Could you check a few things on this drawing? It's one solid part, dimensions in mm from its lowest x, y, z. A direction names the side the tool comes from. Give positions to 0.01 mm unless a question says otherwise; leave off trailing zeros. Loops run counter-clockwise (first coordinate to the right, second up) from the corner with the lowest first, then second, coordinate; pieces in that order, holes last. Notation, with made-up numbers: (62.5, 15.25) - (83.5, 15.25) arc R37 cw to (83.5, 51.25) - close; hole circle Ø3 at (-28, 80). An arc over 180 degrees is marked (long way). Return JSON: item names as keys, results as strings. Group by question number.
(1) On a 3-axis mill with a long thin cutter (end or side, diameter ignored), from which of +Z, -Z, +X, -X, +Y, -Y can I reach the whole of each face in a straight line? I mean the marked faces 1 and 2. Say none if no direction works.
(2) If we section it at B-B (x = 21): Please give me the cut outline in (y, z).
(3) I need wall thicknesses on probe 1 along Y at (x, z) = (5.5, 23); probe 2 along X at (y, z) = (36, 21) (1 decimal). Which ranges of each line are inside material? Lowest first, please. Write a range as [from, to].
(4) If we section it at D-D (z = 39.5): Please give me the cut outline in (x, y), then the cut area to 3 significant figures.
(5) For P1, Ø4, axis at x = 35, y = 22.5, coming from the +Z side; P2, Ø1, axis at y = 22, z = 26.5, coming from the +X side; P3, Ø2.5, axis at x = 5.5, y = 5.5, coming from the +Z side, each with a flat end and sliding along its axis, tell me the tip position at first contact or that it passes through.
(6) If we section it at A-A (z = 22.5): Please give me the cut outline in (x, y).
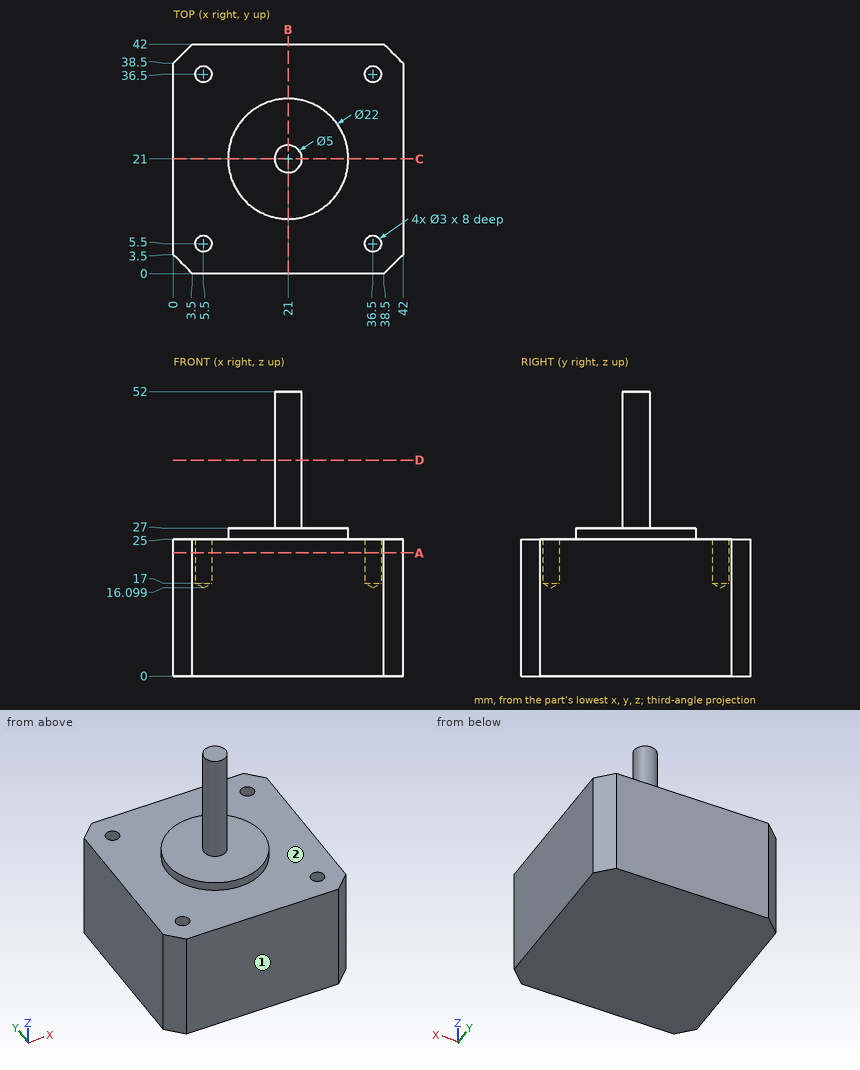
Values:
{
 "1": {"face 1": "+Z, -Z, +X, -X, -Y", "face 2": "+Z"},
 "2": {"outline": "(0, 0) - (42, 0) - (42, 25) - (32, 25) - (32, 27) - (23.5, 27) - (23.5, 52) - (18.5, 52) - (18.5, 27) - (10, 27) - (10, 25) - (0, 25) - close"},
 "3": {"probe 1": "[0, 4], [7, 35], [38, 42]", "probe 2": "[0, 4.1], [6.9, 35.1], [37.9, 42]"},
 "4": {"outline": "circle Ø5 at (21, 21)", "area": "19.6 mm2"},
 "5": {"P1": "z = 25", "P2": "x = 31.99", "P3": "z = 16.85"},
 "6": {"outline": "(0, 3.5) - (3.5, 0) - (38.5, 0) - (42, 3.5) - (42, 38.5) - (38.5, 42) - (3.5, 42) - (0, 38.5) - close; hole circle Ø3 at (5.5, 5.5); hole circle Ø3 at (5.5, 36.5); hole circle Ø3 at (36.5, 5.5); hole circle Ø3 at (36.5, 36.5)"}
}
